Part model, mm, in its own coordinate system. A direction names the side the tool comes from. Coordinates: 2 decimals unless noted, no trailing zeros. Order: outer loops, then holes, each group sorted by start corner. A loop starts at its lowest first (then second) coordinate and runs counter-clockwise, first axis right, second up.
from build123d import *

# Parameters (mm, degrees)
SKETCH1_W           = 53
SKETCH1_H           = 30
BOSS_EXTRUDE1_DEPTH = 2
BOSS_EXTRUDE2_DEPTH = 20


with BuildPart() as part:
    # Sketch1 → Boss-Extrude1 (new body)
    with BuildSketch(Plane(origin=(0, 0, 0), x_dir=(1, 0, 0), z_dir=(0, 1, 0))):
        with Locations((26.5, -15)):
            Rectangle(SKETCH1_W, SKETCH1_H)
    extrude(amount=BOSS_EXTRUDE1_DEPTH)

    # Sketch2 → Boss-Extrude2 (add)
    with BuildSketch(Plane(origin=(0, 2, 0), x_dir=(1, 0, 0), z_dir=(0, 1, 0))):
        Polygon((0, -28), (49, -28), (49, -15), (53, -15), (53, -30), (0, -30), align=None)
        Polygon((49, -2), (0, -2), (0, 0), (53, 0), (53, -6.5), (49, -6.5), align=None)
    extrude(amount=BOSS_EXTRUDE2_DEPTH)


solid = part.part
Q1. Wall check: line 1 along Z through (x, y) = (28, 14); line 2 along X through (y, z) = (10, 3); line 3 along Y through (x, z) = (36.5, 19.5). Give the ranges that are in metal, low to high.
Results list:
line 1: z = 0 to 2, 28 to 30
line 2: x = 49 to 53
line 3: y = 0 to 2
Q2. Pin check, flat tips, straight feed: pin 1 Ø4 at (x, z) = (28.5, 6.5) entering from +Y; pin 2 Ø1.3 at (y, z) = (13.5, 3.5) entering from -X. Stop position of each tip, or through.
Results list:
pin 1: stops at y = 2
pin 2: stops at x = 49
Q3. Mould opens along Z. For faces 4 (the face through (27, 11, 30)), 5 (the face through (26, 11, 0)), 6 (the face through (34, 22, 29)), 7 (the face through (26, 2, 15)) say: pulls with the +Z half, pulls with the -Z half, needs draft (parallel to the pull), parting line crosses it, or undercut.
Results list:
face 4: pulls with the +Z half
face 5: pulls with the -Z half
face 6: needs draft
face 7: undercut
Q4. Cut at A-A on y = 20.25. Write the cut outline in (x, z), and give its area (3 significant figures).
Results list:
outline: (0, 0) - (53, 0) - (53, 6.5) - (49, 6.5) - (49, 2) - (0, 2) - close; (0, 28) - (49, 28) - (49, 15) - (53, 15) - (53, 30) - (0, 30) - close
area: 282 mm2
Q5. Cut at B-B on x = 10.5. Write the cut outline in (y, z).
Results list:
outline: (0, 0) - (22, 0) - (22, 2) - (2, 2) - (2, 28) - (22, 28) - (22, 30) - (0, 30) - close
Q6. Which spindle directions (+Z, -Z, +X, -X, +Y, -Y) get a long thin tool onto all of the face, cutting with end or side? Do faces 1 (the face through (51, 12, 6.5)), 2 (the face through (0, 1, 15)), 3 (the face through (49, 12, 4)). Say none if no direction does.
Results list:
face 1: +X, -X, +Y
face 2: +Z, -Z, -X, +Y, -Y
face 3: -X, +Y
Q7. Cut at C-C on z = 3.5. Write the cut outline in (x, y), and give its area (3 significant figures).
Results list:
outline: (0, 0) - (53, 0) - (53, 22) - (49, 22) - (49, 2) - (0, 2) - close
area: 186 mm2
